Verification items for the finished model (mm, model axes). Face numbers are marked on the shaded views. Give positions to 0.01 mm unless a question says otherwise; leave off trailing zeros. Order: outer loops, then holes, each group sorted by start corner. A loop starts at its lowest first (then second) coordinate and runs counter-clockwise, first axis right, second up. Notation, with made-up numbers: M 66.25,-2 L 94.25,-2 A9 cw 94.25,3 Z; hole C 40.25,29.25 d9. An arc over 180 degrees is marked long. Answer as a JSON object with one key per item and string values.
```python
from build123d import *

# Parameters (mm, degrees)
SKETCH1_R           = 15.875
SKETCH1_R_2         = 3.175
SKETCH1_R_3         = 0.750387242
BOSS_EXTRUDE2_DEPTH = 3.175
SKETCH3_R           = 1.750000056
CUT_EXTRUDE1_DEPTH  = 23.674035261


with BuildPart() as part:
    # Sketch1 → Boss-Extrude2 (new, symmetric)
    with BuildSketch(Plane(origin=(0, 0, 0), x_dir=(1, 0, 0), z_dir=(0, 1, 0))):
        with Locations(Location((0, 0, 0), (0, 0, 270))):
            Circle(SKETCH1_R)
        with Locations(Location((0, 0, 0), (0, 0, 270))):
            Circle(SKETCH1_R_2, mode=Mode.SUBTRACT)
        with Locations(Location((9.525, 0, 0), (0, 0, 270))):
            Circle(SKETCH1_R_3, mode=Mode.SUBTRACT)
        with Locations(Location((-4.7625, -8.248891971, 0), (0, 0, 270))):
            Circle(SKETCH1_R_3, mode=Mode.SUBTRACT)
        with Locations(Location((-4.7625, 8.248891971, 0), (0, 0, 270))):
            Circle(SKETCH1_R_3, mode=Mode.SUBTRACT)
    extrude(amount=BOSS_EXTRUDE2_DEPTH, both=True)

    # Sketch3 → Cut-Extrude1 (cut, through all)
    with BuildSketch(Plane(origin=(0, 0, 0), x_dir=(0, 0, -1), z_dir=(1, 0, 0))):
        Circle(SKETCH3_R)
    extrude(amount=-CUT_EXTRUDE1_DEPTH, mode=Mode.SUBTRACT)


solid = part.part
```
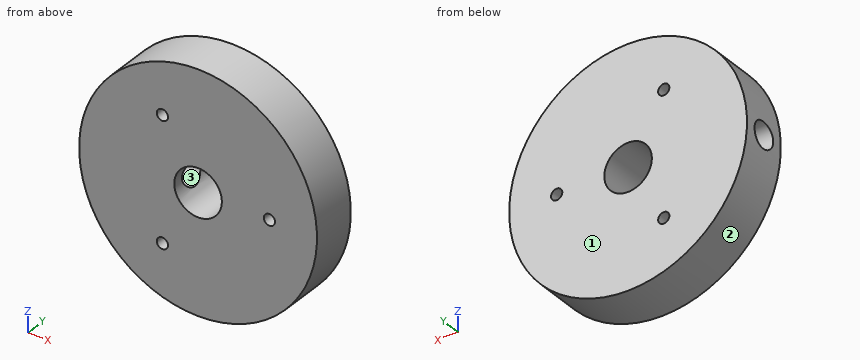
Q1. Section check A-A on x = 0. Record the cut outline in (y, z) (3 decimals), then the cut area to 3 significant figures.
Resolved:
{"outline": "M -3.175,-15.875 L 3.175,-15.875 L 3.175,-3.175 L -3.175,-3.175 Z; M -3.175,3.175 L 3.175,3.175 L 3.175,15.875 L -3.175,15.875 Z", "area": "161 mm²"}
Q2. Section check B-B on z = 0. Record the cut outline in (x, y) (3 decimals).
Resolved:
{"outline": "M -15.875,-3.175 L -3.175,-3.175 L -3.175,-1.75 L -15.875,-1.75 Z; M -15.875,1.75 L -3.175,1.75 L -3.175,3.175 L -15.875,3.175 Z; M 3.175,-3.175 L 8.775,-3.175 L 8.775,3.175 L 3.175,3.175 Z; M 10.275,-3.175 L 15.875,-3.175 L 15.875,3.175 L 10.275,3.175 Z"}
Q3. Release check for a two-part mould opening along Z. For the marked faces 1, 2 and 3 record: +Z half, -Z half, draft (parallel to the pull), parting line (faces both ways), or undercut.
Resolved:
{"face 1": "draft", "face 2": "parting line", "face 3": "undercut"}
Q4. Section check C-C on y = -0.75. Count the separate pieces of the cut face and the enclosed holes in it, then the cut area to 3 significant figures.
Resolved:
{"separate pieces": "1", "enclosed holes": "3", "area": "714 mm²"}
Q5. Gauge pin test, flat ends, axial feed: pin 1 Ø3 at (y, z) = (0, 0) entering from -X; pin 2 Ø3 at (x, y) = (-12, -1) entering from +Z; pin 3 Ø4 at (x, z) = (0, 0) entering from -Y; pin 4 Ø2 at (x, y) = (-1.5, 2.5) entering from -Z. Record the tip position at first contact, or that the pin passes through.
Resolved:
{"pin 1": "stops at x = 2.8", "pin 2": "stops at z = 11.91", "pin 3": "passes through", "pin 4": "stops at z = -15.87"}
Q6. Material ranges on L1, parallel to X at y = 2.25, z = 0 (3 decimals); L2, parallel to X at y = 0.75, z = 0 (3 decimals); L3, parallel to Z at x = -9, y = -1, recorded low to high.
Resolved:
{"L1": "x = -15.875 to -3.175, 3.175 to 8.775, 10.275 to 15.875", "L2": "x = 3.175 to 8.775, 10.275 to 15.875", "L3": "z = -13.08 to -1.44, 1.44 to 13.08"}
